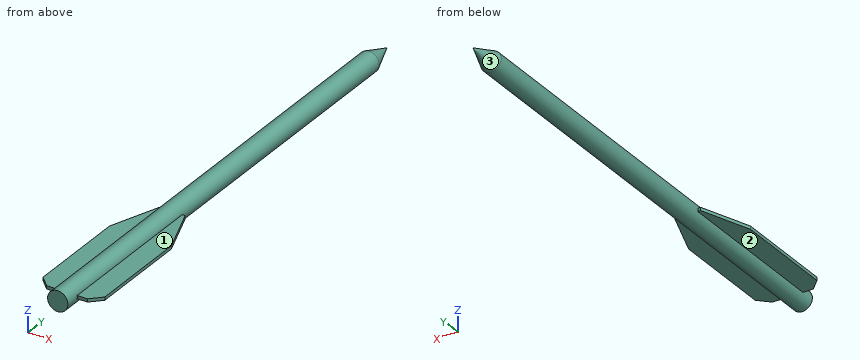
```python
from build123d import *

# Parameters (mm, degrees)
SKETCH1_R           = 3.2
BOSS_EXTRUDE1_DEPTH = 161
CHAMFER1_SIZE       = 3.2
CHAMFER1_SIZE2      = 8.791927742
FLETCHING_DEPTH     = 0.5


with BuildPart() as part:
    # Sketch1 → Boss-Extrude1 (new body)
    with BuildSketch(Plane(origin=(0, 0, 0), x_dir=(1, 0, 0), z_dir=(0, 1, 0))):
        with Locations(Location((0, 0, 0), (0, 0, 270))):
            Circle(SKETCH1_R)
    extrude(amount=BOSS_EXTRUDE1_DEPTH)

    # Chamfer1
    chamfer1_edges = [part.edges().sort_by_distance(p)[0] for p in [
        (0, 161, -3.2),
    ]]
    chamfer1_side = [part.faces().sort_by_distance(p)[0] for p in [
        (0, 161, 0),
    ]]
    chamfer(chamfer1_edges, length=CHAMFER1_SIZE, length2=CHAMFER1_SIZE2, reference=chamfer1_side[0])

    # Sketch2 → Fletching (add, symmetric)
    with BuildSketch(Plane.XY):
        Polygon((0, 4.6), (-6.45, 4.6), (-9.75, 7.9), (-9.75, 40.425060307), (-4.081185551, 56), (0, 56), align=None)
    fletching = extrude(amount=FLETCHING_DEPTH, both=True)

    # Fletchings: Fletching across plane
    add(fletching.mirror(Plane(origin=(0, 0, 0), x_dir=(0, 0, 1), z_dir=(1, 0, 0))))


solid = part.part
```
Design review of the part built by this model. Coordinates are the model's own, in mm. Face numbers are marked on the shaded views. A direction names the side the tool comes from. Coordinates: 2 decimals unless noted, no trailing zeros. Write each loop counter-clockwise with the first axis right and the second up, starting at its lowest first coordinate (ties: lowest second). Pieces come first, ordered by that corner, then holes.
1) Insertion check: pin 1 (7 mm diameter, centred on x = -5.5, y = 19.5, fed in from -Z); pin 2 (3 mm diameter, centred on x = 3, y = 133.5, fed in from -Z); pin 3 (2 mm diameter, centred on x = 7.5, y = 37.5, fed in from -Z). Each pin has a flat end and moves straight along its axis. Give the tip position at first contact, or say it passes through.
2) Add section A-A (y = 21). Write out the cut boundary in (x, z).
3) Add section B-B (y = 96.5). Write out the cut boundary in (x, z), plus the area to 3 significant figures.
4) To check wall thickness, follow L1, parallel to Z at x = 7.5, y = 44.5; L2, parallel to X at y = 136, z = 0; L3, parallel to Y at x = 0.25, z = -0.5. State the ranges of each line that lie inside material, in increasing order.
5) Machinability: for the marked faces 1, 2 and 3, which of the approach directions +Z, -Z, +X, -X, +Y, -Y give a long, thin tool a straight path to every point of the face, cutting with its end or side? Answer none if there is none.
Check result:
1. pin 1: stops at z = -2.5
1. pin 2: stops at z = -2.83
1. pin 3: stops at z = -0.5
2. outline: (-9.75, -0.5) - (-3.16, -0.5) arc R3.2 ccw to (3.16, -0.5) - (9.75, -0.5) - (9.75, 0.5) - (3.16, 0.5) arc R3.2 ccw to (-3.16, 0.5) - (-9.75, 0.5) - close
3. outline: circle Ø6.4 at (0, 0)
3. area: 32.2 mm2
4. L1: z = -0.5 to 0.5
4. L2: x = -3.2 to 3.2
4. L3: y = 0 to 159.46
5. face 1: +Z, +X, +Y, -Y
5. face 2: -Z, -X, +Y, -Y
5. face 3: +Y
